For this review, take the finished solid that the model builds, in its own axes (mm). A direction names the side the tool comes from. Give positions to 0.01 mm unless a question says otherwise; leave off trailing zeros. Loops run counter-clockwise (first coordinate to the right, second up) from the corner with the lowest first, then second, coordinate; pieces in that order, holes last.
```python
from build123d import *

# Parameters (mm, degrees)
SZKIC1_W                    = 39
SZKIC1_H                    = 178.7
DODANIE_WYCI_GNI_CIE1_DEPTH = 6
WYTNIJ_WYCI_GNI_CIE1_DEPTH  = 208.642171135
WYTNIJ_WYCI_GNI_CIE2_DEPTH  = 208.642171135
SZYK_LINIOWY1_COUNT         = 2
SZYK_LINIOWY1_PITCH         = 90
SZYK_LINIOWY2_COUNT         = 2
SZYK_LINIOWY2_PITCH         = 23.9
SZKIC4_W                    = 6
SZKIC4_H                    = 6
DODANIE_WYCI_GNI_CIE2_DEPTH = 5.8


with BuildPart() as part:
    # Szkic1 → Dodanie-wyciągnięcie1 (new body)
    with BuildSketch(Plane.XY):
        with Locations((-35.991181586, -110.65)):
            Rectangle(SZKIC1_W, SZKIC1_H)
    extrude(amount=-DODANIE_WYCI_GNI_CIE1_DEPTH)

    # Szkic2 → Wytnij-wyciągnięcie1 (cut, through all)
    with BuildSketch(Plane(origin=(0, 0, -6), x_dir=(-1, 0, 0), z_dir=(0, 0, -1))):
        Polygon((16.491181586, -160), (16.491181586, -156.9), (20.491181586, -156.9), (20.491181586, -155.525), (22.491181586, -155.525), (22.491181586, -156.9), (22.991181586, -156.9), (22.991181586, -160), (22.491181586, -160), (22.491181586, -161.375), (20.491181586, -161.375), (20.491181586, -160), align=None)
    wytnij_wyci_gni_cie1 = extrude(amount=-WYTNIJ_WYCI_GNI_CIE1_DEPTH, mode=Mode.SUBTRACT)

    # Szkic3 → Wytnij-wyciągnięcie2 (cut, through all)
    with BuildSketch(Plane(origin=(0, 0, -6), x_dir=(-1, 0, 0), z_dir=(0, 0, -1))):
        Polygon((49.491181586, -200), (49.491181586, -196), (50.866181586, -196), (50.866181586, -194), (49.491181586, -194), (49.491181586, -193.5), (46.391181586, -193.5), (46.391181586, -194), (45.016181586, -194), (45.016181586, -196), (46.391181586, -196), (46.391181586, -200), align=None)
    wytnij_wyci_gni_cie2 = extrude(amount=-WYTNIJ_WYCI_GNI_CIE2_DEPTH, mode=Mode.SUBTRACT)

    # Szyk liniowy1: Wytnij-wyciągnięcie1 ×2
    with Locations(*[(0, i * SZYK_LINIOWY1_PITCH, 0) for i in range(1, SZYK_LINIOWY1_COUNT)]):
        add(wytnij_wyci_gni_cie1, mode=Mode.SUBTRACT)

    # Szyk liniowy2: Wytnij-wyciągnięcie2 ×2
    with Locations(*[(i * SZYK_LINIOWY2_PITCH, 0, 0) for i in range(1, SZYK_LINIOWY2_COUNT)]):
        add(wytnij_wyci_gni_cie2, mode=Mode.SUBTRACT)

    # Szkic4 → Dodanie-wyciągnięcie2 (add)
    with BuildSketch(Plane(origin=(0, -21.3, 0), x_dir=(1, 0, 0), z_dir=(0, 1, 0))):
        with Locations((-52.491181586, 3)):
            Rectangle(SZKIC4_W, SZKIC4_H)
    extrude(amount=DODANIE_WYCI_GNI_CIE2_DEPTH)


solid = part.part
```
Q1. Machinability: for faces 5 (the flat face through (-16.491, -114, -3)), 6 (the flat face through (-22.491, -198, -3)), 7 (the flat face through (-18, -156.9, -3)), which of the approach directions +Z, -Z, +X, -X, +Y, -Y give a long, thin tool a straight path to every point of the face, cutting with its end or side? Answer none if there is none.
Answers:
face 5: +Z, -Z, +X, +Y, -Y
face 6: +Z, -Z, -Y
face 7: +Z, -Z, +X
Q2. Mouldability with a two-part tool opening along X and no side actions: class faces 1 (the flat face through (-49.491, -198, -3)), 2 (the flat face through (-25.591, -198, -3)), 3 (the flat face through (-33, -21.3, -3)), 4 (the flat face through (-49.491, -18, -3)) as +X half, -X half, draft (parallel to the pull), parting line (faces both ways), or undercut.
Answers:
face 1: undercut
face 2: undercut
face 3: draft
face 4: +X half
Q3. For probe 1 along Y at (x, z) = (-50, -5); probe 2 along Y at (x, z) = (-43, -1.55), list the stretches that pass through material, from the lowest coordinate up.
Answers:
probe 1: y = -200 to -196, -194 to -15.5
probe 2: y = -200 to -21.3
Q4. Consider section A-A on x = -38.5. Give the boundary of the cut face in (y, z).
Answers:
outline: (-200, -6) - (-21.3, -6) - (-21.3, 0) - (-200, 0) - close
Q5. For pin 1 Ø0.9 at (x, z) = (-48.5, -2) entering from -Y; pin 2 Ø1.5 at (x, z) = (-22.5, -1) entering from +Y, all flat-tipped, find the tip position at first contact; note any pin that passes through.
Answers:
pin 1: stops at y = -193.5
pin 2: stops at y = -21.3
